Autodesk Fusion 360 part; units mm, degrees
sketch "Sketch1" plane through (0, 0, 0) normal (0, 0, 1) x (1, 0, 0)
  line L0 (11.5, 4) -> (-11.5, 4)
  line L1 (-11.5, 4) -> (-11.5, -4)
  line L2 (-11.5, -4) -> (11.5, -4)
  line L3 (11.5, -4) -> (11.5, 4)
  line L4 (11.5, 4) -> (-11.5, -4) construction
  line L5 (-11.5, 4) -> (11.5, -4) construction
  line L6 (-11.5, 4) -> (11.5, 4)
  line L7 (11.5, 4) -> (11.5, 2.4)
  line L8 (11.5, 2.4) -> (-11.5, 2.4)
  line L9 (-11.5, 2.4) -> (-11.5, 4)
  dimension "d1" = 23
  dimension "d2" = 8
  dimension "d3" = 1.6
extrude "Extrude1" add sketch "Sketch1" along normal blind 1.6
extrude "Extrude2" add sketch "Sketch1" along normal blind 15 contours L0 L1 L3 L6 L7 L8 L9
hole "Hole1" at (-6.5, 2.4, 10) direction (0, 1, 0) diameter 3.4 depth 9 tip angle 118
hole "Hole2" at (6.5, 2.4, 10) direction (0, 1, 0) diameter 3.4 depth 12 tip angle 118
sketch "Sketch2" plane through (0, 0, 0) normal (1, 0, 0) x (0, 1, 0)
  line L0 (2.4, 1.6) -> (-4, 1.6)
  line L1 (-4, 1.6) -> (2.4, 1.6)
  line L2 (2.4, 1.6) -> (2.4, 15)
  line L3 (-3.1915, 1.6) -> (2.4, 7.2966)
  line L4 (2.4, 1.6) -> (-3.1915, 1.6)
extrude "Extrude3" add sketch "Sketch2" along normal blind 1.6 from surface at -9.6
extrude "Extrude4" add sketch "Sketch2" along normal blind 1.6 from surface at -0.8
extrude "Extrude5" add sketch "Sketch2" along normal blind 1.6 from surface at 8
Here's how the part is built. I have some questions about the finished solid (model axes, mm). A direction names the side the tool comes from. Give positions to 0.01 mm unless a question says otherwise; leave off trailing zeros. Loops run counter-clockwise (first coordinate to the right, second up) from the corner with the lowest first, then second, coordinate; pieces in that order, holes last. Notation, with made-up numbers: M 29.5,10.25 L 67.5,10.25 A33 ccw 67.5,46.25 Z; hole C 1.25,29.5 d5. An arc over 180 degrees is marked long. Use one line per item in the form item = value. Start each with the question number.
Q1. Thinking about a two-plate mould opening in Z: for faces 1 (the flat face through (11.5, 3, 5)), 2 (the cylindrical face through (8, 3.2, 9.2)), 3 (the flat face through (-8.811, -0.435, 4.408)), 4 (the cylindrical face through (-5, 3.2, 9.2)), which applies, +Z half, -Z half, draft (parallel to the pull), parting line (faces both ways), or undercut?
Q2. Which directions (+Z, -Z, +X, -X, +Y, -Y) give clear straight access to the entire face, cutting with the end or side of a thin tool? Please do faces 5 (the flat face through (-9.6, 1, 3)), 6 (the flat face through (8, 1, 3)), 7 (the flat face through (9.6, 1, 3)), 8 (the flat face through (-11.5, 3, 5)).
Q3. I need wall thicknesses on line 1 along X through (y, z) = (3.2, 10); line 2 along X through (y, z) = (-1, 2.5); line 3 along Z through (x, y) = (6.5, 3.15). Which ranges of each line are inside material? Lowest first, please.
Q4. If we section it at A-A (x = -6.5): Write out the boundary of the cut face in (y, z).
Q5. Will these pins go through, and if not, where does the flat tip stop? pin 1 Ø1.7 at (y, z) = (0.5, 3.5) entering from +X; pin 2 Ø2.5 at (x, z) = (-6.5, 10) entering from +Y; pin 3 Ø8 at (x, z) = (5.5, 12) entering from -Y; pin 4 Ø3 at (y, z) = (-0.5, 5.5) entering from -X.
Q6. If we section it at B-B (z = 10): Write out the boundary of the cut face in (x, y), then the cut area to 3 significant figures.
Q7. If we section it at D-D (y = 1.5): Write out the boundary of the cut face in (x, z), then the cut area to 3 significant figures.
Q8. If we section it at C-C (x = 9): Write out the boundary of the cut face in (y, z), then the cut area to 3 significant figures.
Taken from the geometry:
q1.face_1 = draft
q1.face_2 = undercut
q1.face_3 = +Z half
q1.face_4 = undercut
q2.face_5 = +Z, -X, -Y
q2.face_6 = +Z, -Y
q2.face_7 = +Z, +X, -Y
q2.face_8 = +Z, -Z, -X, +Y, -Y
q3.line_1 = -11.5 to -8.2, -4.8 to 4.8, 8.2 to 11.5
q3.line_2 = -9.6 to -8, -0.8 to 0.8, 8 to 9.6
q3.line_3 = 0 to 8.3, 11.7 to 15
q4.outline = M -4,0 L 4,0 L 4,8.3 L 2.4,8.3 L 2.4,1.6 L -4,1.6 Z; M 2.4,11.7 L 4,11.7 L 4,15 L 2.4,15 Z
q5.pin_1 = 9.6
q5.pin_2 = through
q5.pin_3 = 2.4
q5.pin_4 = -9.6
q6.outline = M -11.5,2.4 L -8.2,2.4 L -8.2,4 L -11.5,4 Z; M -4.8,2.4 L 4.8,2.4 L 4.8,4 L -4.8,4 Z; M 8.2,2.4 L 11.5,2.4 L 11.5,4 L 8.2,4 Z
q6.area = 25.9 mm^2
q7.outline = M -11.5,0 L 11.5,0 L 11.5,1.6 L 9.6,1.6 L 9.6,6.38 L 8,6.38 L 8,1.6 L 0.8,1.6 L 0.8,6.38 L -0.8,6.38 L -0.8,1.6 L -8,1.6 L -8,6.38 L -9.6,6.38 L -9.6,1.6 L -11.5,1.6 Z
q7.area = 59.7 mm^2
q8.outline = M -4,0 L 4,0 L 4,15 L 2.4,15 L 2.4,7.3 L -3.19,1.6 L -4,1.6 Z
q8.area = 50.2 mm^2
